from build123d import *

# Parameters (mm, degrees)
SKETCH2_R                        = 22.225
BOSS_EXTRUDE1_DEPTH              = 25.4
F_1_4_1_5_DIAMETER_HOLE1_D       = 38.1
F_1_4_1_5_DIAMETER_HOLE1_DEPTH   = 3.302
F_1_4_1_5_DIAMETER_HOLE2_D       = 38.1
F_1_4_1_5_DIAMETER_HOLE2_DEPTH   = 3.302
F_1_4_0_125_DIAMETER_HOLE1_D     = 3.175
F_1_4_0_125_DIAMETER_HOLE1_DEPTH = 16.002
F_1_4_0_125_DIAMETER_HOLE1_TIP   = 0.953866233


with BuildPart() as part:
    # Sketch2 → Boss-Extrude1 (new body)
    with BuildSketch(Plane(origin=(0, 0, 0), x_dir=(1, 0, 0), z_dir=(0, 1, 0))):
        Circle(SKETCH2_R)
    extrude(amount=BOSS_EXTRUDE1_DEPTH)

    # 1/4 (1.5) Diameter Hole1
    with Locations(Plane(origin=(0, 25.4, 0), x_dir=(1, 0, 0), z_dir=(0, 1, 0))):
        with Locations((0, 0)):
            Hole(F_1_4_1_5_DIAMETER_HOLE1_D / 2, depth=F_1_4_1_5_DIAMETER_HOLE1_DEPTH)

    # 1/4 (1.5) Diameter Hole2
    with Locations(Plane(origin=(0, 0, 0), x_dir=(-1, 0, 0), z_dir=(0, -1, 0))):
        with Locations((0, 0)):
            Hole(F_1_4_1_5_DIAMETER_HOLE2_D / 2, depth=F_1_4_1_5_DIAMETER_HOLE2_DEPTH)

    # 1/4 (0.125) Diameter Hole1
    with Locations(Plane.XY.offset(22.225)):
        with Locations((0, 12.7)):
            Hole(F_1_4_0_125_DIAMETER_HOLE1_D / 2, depth=F_1_4_0_125_DIAMETER_HOLE1_DEPTH)
            with Locations((0, 0, -(F_1_4_0_125_DIAMETER_HOLE1_DEPTH + F_1_4_0_125_DIAMETER_HOLE1_TIP / 2))):  # 118° drill point
                Cone(0, F_1_4_0_125_DIAMETER_HOLE1_D / 2, F_1_4_0_125_DIAMETER_HOLE1_TIP, mode=Mode.SUBTRACT)


solid = part.part
Input: part model. Units: mm. Frame: model coordinates. A direction names the side the tool comes from. Coordinates: 2 decimals unless noted, no trailing zeros. Order: outer loops, then holes, each group sorted by start corner. A loop starts at its lowest first (then second) coordinate and runs counter-clockwise, first axis right, second up. Notation, with made-up numbers: M -17.5,88.5 L 25.5,88.5 A22 ccw 25.5,94.5 Z; hole C -15.75,-1.5 d7. An arc over 180 degrees is marked long. Write item = value, one per line. Start each with the question number.
(1) Section A-A on z = 10. Output: boundary loops of the cut face in (x, y) (1 decimal), and give its area (3 significant figures).
(2) Reachability of faces 5 (the flat face through (16.4, 0, -10)), 6 (the flat face through (0, 3.302, 0)), 7 (the cylindrical face through (0.207, 14.274, 14.113)), 8 (the cylindrical face through (15.12, 23.73, 11.59)) from +Z, -Z, +X, -X, +Y, -Y: full face, straight path, thin tool, end or side. Return the list, or none.
(3) Pull-direction query (X, two-part tool) for faces 1 (the conical face through (-0.036, 12.973, 5.435)), 2 (the cylindrical face through (21.199, 12.522, -6.676)), 3 (the flat face through (0, 22.098, 0)), 4 (the flat face through (16.4, 25.4, -10)); classes: released by +X, released by -X, zero draft, split by the parting line, or undercut.
(4) Section D-D on y = 9.5. Output: boundary loops of the cut face in (x, z) (3 decimals).
(5) Line query: line 1 along Z through (x, y) = (0, 2.2) (3 decimals); line 2 along Y through (x, z) = (0, 13); line 3 along Y through (x, z) = (8.5, 8). Output: solid intervals per line, ascending. Write a range as [from, to].
(6) Section B-B on z = 0. Output: boundary loops of the cut face in (x, y) (3 decimals).
(7) First-contact query: P1, Ø1, axis at x = -2.5, y = 9, coming from the -Z side; P2, Ø2, axis at x = 2.5, z = -2.5, coming from the -Y side; P3, Ø4, axis at x = 3, y = 10, coming from the -Z side. Flat tips, straight axial feed; report the tip coordinate or a pass-through.
(8) Section C-C on x = 5.5. Output: boundary loops of the cut face in (y, z), and give its area (3 significant figures).
Result set:
q1.outline = M -19.8,0 L -16.2,0 L -16.2,3.3 L 16.2,3.3 L 16.2,0 L 19.8,0 L 19.8,25.4 L 16.2,25.4 L 16.2,22.1 L -16.2,22.1 L -16.2,25.4 L -19.8,25.4 Z; hole C 0,12.7 d3.2
q1.area = 786 mm²
q2.face_5 = +Z, -Z, +X, -X, -Y
q2.face_6 = -Y
q2.face_7 = +Z
q2.face_8 = +Y
q3.face_1 = undercut
q3.face_2 = split by the parting line
q3.face_3 = undercut
q3.face_4 = zero draft
q4.outline = C 0,0 d44.45
q5.line_1 = [-22.225, -19.05], [19.05, 22.225]
q5.line_2 = [3.3, 11.11], [14.29, 22.1]
q5.line_3 = [3.3, 22.1]
q6.outline = M -22.225,0 L -19.05,0 L -19.05,3.302 L 19.05,3.302 L 19.05,0 L 22.225,0 L 22.225,25.4 L 19.05,25.4 L 19.05,22.098 L -19.05,22.098 L -19.05,25.4 L -22.225,25.4 Z
q7.P1 = -22.13
q7.P2 = 3.3
q7.P3 = -22.2
q8.outline = M 0,-21.53 L 25.4,-21.53 L 25.4,-18.24 L 22.1,-18.24 L 22.1,18.24 L 25.4,18.24 L 25.4,21.53 L 0,21.53 L 0,18.24 L 3.3,18.24 L 3.3,-18.24 L 0,-18.24 Z
q8.area = 853 mm²
